```python
from build123d import *

# Parameters (mm, degrees)
BOSS_EXTRUDE1_DEPTH = 1.5


with BuildPart() as part:
    # Sketch3 → Boss-Extrude1 (new body, symmetric)
    with BuildSketch(Plane(origin=(0, 0, 0), x_dir=(1, 0, 0), z_dir=(0, 1, 0))):
        with BuildLine():
            Line((6.39, 1.715), (-6.39, 1.715))
            ThreePointArc((-6.39, 1.715), (-8.334543648, 2.520456352), (-9.14, 4.465))
            Line((-9.14, 4.465), (-9.14, 5.925))
            Line((-9.14, 5.925), (-10.75, 5.925))
            Line((-10.75, 5.925), (-10.75, -2.428885313))
            Line((-10.75, -2.428885313), (-9.053324958, -2.428885313))
            ThreePointArc((-9.053324958, -2.428885313), (-8.483744199, -2.513924788), (-7.963842259, -2.761626073))
            ThreePointArc((-7.963842259, -2.761626073), (-7.358164616, -3.457324711), (-7.14, -4.353564747))
            Line((-7.14, -4.353564747), (-7.14, -5.925))
            Line((-7.14, -5.925), (7.14, -5.925))
            Line((7.14, -5.925), (7.14, -4.353564747))
            ThreePointArc((7.14, -4.353564747), (7.358164616, -3.457324711), (7.963842259, -2.761626073))
            ThreePointArc((7.963842259, -2.761626073), (8.483744199, -2.513924788), (9.053324958, -2.428885313))
            Line((9.053324958, -2.428885313), (10.75, -2.428885313))
            Line((10.75, -2.428885313), (10.75, 5.925))
            Line((10.75, 5.925), (9.14, 5.925))
            Line((9.14, 5.925), (9.14, 4.465))
            ThreePointArc((9.14, 4.465), (8.334543648, 2.520456352), (6.39, 1.715))
        make_face()
    extrude(amount=BOSS_EXTRUDE1_DEPTH, both=True)


solid = part.part
```
Check sheet for the modelled part. Datum: model origin and axes. Units: mm. A direction names the side the tool comes from. Give positions to 0.01 mm unless a question says otherwise; leave off trailing zeros. Order: outer loops, then holes, each group sorted by start corner. A loop starts at its lowest first (then second) coordinate and runs counter-clockwise, first axis right, second up. Notation, with made-up numbers: (41.25, -22.75) -> (89.25, -22.75) arc R20 ccw to (89.25, -4.75) -> close; hole circle Ø7 at (-31, 1.25). An arc over 180 degrees is marked (long way). Return JSON: item names as keys, results as strings.
1. Cross-section at B-B, the plane y = 1.15. Record the cut outline in (x, z) (3 decimals).
From the geometry:
{"outline": "(-10.75, -5.925) -> (-9.14, -5.925) -> (-9.14, -4.465) arc R2.75 cw to (-6.39, -1.715) -> (6.39, -1.715) arc R2.75 cw to (9.14, -4.465) -> (9.14, -5.925) -> (10.75, -5.925) -> (10.75, 2.429) -> (9.053, 2.429) arc R1.95 cw to (7.964, 2.762) arc R1.95 cw to (7.14, 4.354) -> (7.14, 5.925) -> (-7.14, 5.925) -> (-7.14, 4.354) arc R1.95 cw to (-7.964, 2.762) arc R1.95 cw to (-9.053, 2.429) -> (-10.75, 2.429) -> close"}
2. Cross-section at C-C, the plane x = 9.5. Record the cut outline in (y, z) (3 decimals), plus the area to 3 significant figures.
From the geometry:
{"outline": "(-1.5, -5.925) -> (1.5, -5.925) -> (1.5, 2.429) -> (-1.5, 2.429) -> close", "area": "25.1 mm^2"}
3. Material ranges on probe 1 along X at (y, z) = (0.1, -2.75); probe 2 along X at (y, z) = (1.1, -5.5); probe 3 along X at (y, z) = (0.05, 4.5), recorded low to high. Write a range as [from, to].
From the geometry:
{"probe 1": "[-10.75, -8.54], [8.54, 10.75]", "probe 2": "[-10.75, -9.14], [9.14, 10.75]", "probe 3": "[-7.14, 7.14]"}
4. Cross-section at D-D, the plane z = 3.5. Record the cut outline in (x, y), plus the area to 3 significant figures.
From the geometry:
{"outline": "(-7.34, -1.5) -> (7.34, -1.5) -> (7.34, 1.5) -> (-7.34, 1.5) -> close", "area": "44.0 mm^2"}
5. Set-up check for faces 1 (the cylindrical face through (-8.313, 0.021, -2.499)), 2 (the flat face through (10, 0, 2.429)), 3 (the flat face through (-10, 0, 2.429)), 4 (the flat face through (10.75, 0, -2)), 5 (the flat face through (0, 1.5, 1)): record each of +Z, -Z, +X, -X, +Y, -Y from which the full face is reachable in a straight line by a thin tool's end or side.
From the geometry:
{"face 1": "-Z, +Y, -Y", "face 2": "+Z, +X, +Y, -Y", "face 3": "+Z, -X, +Y, -Y", "face 4": "+Z, -Z, +X, +Y, -Y", "face 5": "+Z, -Z, +X, -X, +Y"}
6. Go/stop test with flat-tipped pins: P1, Ø1.3, axis at y = -0.5, z = 5, coming from the -X side; P2, Ø0.8, axis at y = 0.5, z = 5, coming from the +X side; P3, Ø0.5, axis at x = -9.5, y = 0.5, coming from the +Z side. Record where each tip stops, or that it passes through.
From the geometry:
{"P1": "x = -7.14", "P2": "x = 7.14", "P3": "z = 2.43"}
7. Cross-section at A-A, the plane z = -3. Record the cut outline in (x, y), plus the area to 3 significant figures.
From the geometry:
{"outline": "(-10.75, -1.5) -> (-8.72, -1.5) -> (-8.72, 1.5) -> (-10.75, 1.5) -> close; (8.72, -1.5) -> (10.75, -1.5) -> (10.75, 1.5) -> (8.72, 1.5) -> close", "area": "12.2 mm^2"}
